Autodesk Inventor part; units mm, degrees
ref_plane "YZ Plane" through (0, 0, 0) normal (1, 0, 0) x (0, 1, 0)
ref_plane "XZ Plane" through (0, 0, 0) normal (0, 1, 0) x (-1, 0, 0)
ref_plane "XY Plane" through (0, 0, 0) normal (0, 0, 1) x (1, 0, 0)
sketch "Skizze1" plane through (0, 0, 0) normal (0, 0, 1) x (1, 0, 0)
  line L0 (16.6415, 9.8457) -> (8.5751, 9.8457)
  line L1 (8.5751, 9.8457) -> (8.5751, -9.8457)
  line L2 (8.5751, -9.8457) -> (16.6415, -9.8457)
  line L3 (16.6415, -9.8457) -> (16.6415, 9.8457)
  line L4 (16.6415, 9.8457) -> (8.5751, -9.8457) construction
  line L5 (8.5751, 9.8457) -> (16.6415, -9.8457) construction
  circle A0 centre (12.6083, 0) radius 2.6
  point P0 (0, 0)
  dimension "d0" = 5.2
extrude "Extrusion1" add sketch "Skizze1" along normal blind 3
sketch "Skizze2" plane through (0, 0, 3) normal (0, 0, 1) x (1, 0, 0)
  circle A0 centre (12.6083, 0) radius 2.6 construction
  line L0 (16.6415, 9.8457) -> (8.5751, 9.8457) construction
  line L1 (8.5751, 9.8457) -> (8.5751, -9.8457) construction
  line L2 (8.5751, -9.8457) -> (16.6415, -9.8457) construction
  line L3 (16.6415, -9.8457) -> (16.6415, 9.8457) construction
  line L4 (8.5751, 9.8457) -> (8.5751, -9.8457)
  line L5 (16.6415, -9.8457) -> (8.5751, -9.8457)
  line L6 (8.5751, -9.8457) -> (8.5751, -6.7929)
  line L7 (8.5751, -6.7929) -> (16.6415, -6.7929)
  line L8 (16.6415, -6.7929) -> (16.6415, -9.8457)
  line L9 (16.6415, -9.8457) -> (16.6415, 9.8457)
  line L10 (8.5751, 9.8457) -> (16.6415, 9.8457)
  line L11 (16.6415, 9.8457) -> (16.6415, 7.3365)
  line L12 (16.6415, 7.3365) -> (8.5751, 7.3365)
  line L13 (8.5751, 7.3365) -> (8.5751, 9.8457)
  point P0 (0, 0)
extrude "Extrusion2" add sketch "Skizze2" along normal blind 25 contours L10 L9 L12 L4 | L7 L8 L5 L4
sketch "Skizze3" plane through (8.5751, 7.3365, 3) normal (0, -1, 0) x (1, 0, 0)
  line L0 (8.0665, 0) -> (0, 0)
  line L1 (8.0665, 0) -> (8.0665, 25)
  line L2 (0, 25) -> (8.0665, 25)
  line L3 (0, 0) -> (0, 25)
  circle A0 centre (4.0332, 20.469) radius 1.4552
  point P0 (-8.5751, -3)
extrude "Extrusion3" cut sketch "Skizze3" along normal through all both and the other way through all contours A0
sketch "Skizze4" plane through (8.5751, -9.8457, 0) normal (0, -1, 0) x (1, 0, 0)
  line L0 (8.0665, 3) -> (8.0665, 28)
  line L1 (0, 3) -> (0, 28)
  line L2 (8.0665, 28) -> (0, 28)
  line L3 (0, 28) -> (0, 26.1511)
  line L4 (0, 26.1511) -> (8.0665, 26.1511)
  line L5 (8.0665, 26.1511) -> (8.0665, 28)
  point P0 (-8.5751, 0)
extrude "Extrusion4" cut sketch "Skizze4" against normal through all
sketch "Skizze5" plane through (16.6415, -9.8457, 0) normal (1, 0, 0) x (0, 0, -1)
  ellipse E0 centre (-12.9855, 10.4116) end of major axis (-22.9331, 10.4116) minor radius 7.8919
  point P0 (0, 9.8457)
extrude "Extrusion5" cut sketch "Skizze5" along normal through all both and the other way through all
properties part number "amt_dragster"
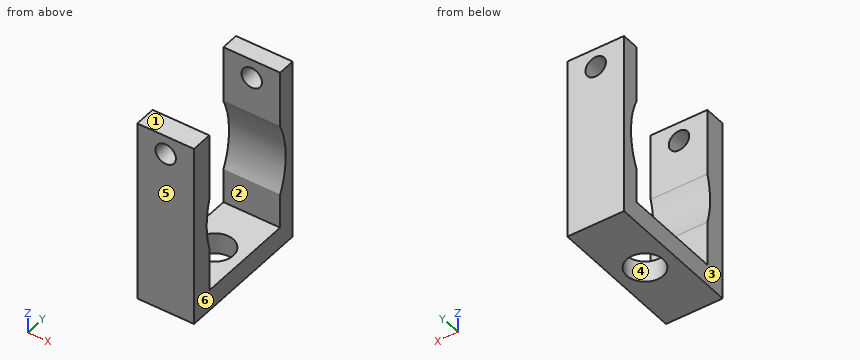
Work out the finished part from the listing and answer in its coordinate system (mm). Face numbers are marked on the shaded views. A direction names the side the tool comes from. Round coordinates to 2 decimals unless told otherwise and drop trailing zeros. Order: outer loops, then holes, each group sorted by start corner. A loop starts at its lowest first (then second) coordinate and runs counter-clockwise, first axis right, second up.
Q1. The mould has two halves that part along X. Classify the marked faces 3, 4, 5 and 6: pulls with the +X half, pulls with the -X half, needs draft (parallel to the pull), parting line crosses it, or undercut.
Solution:
face 3: pulls with the -X half
face 4: undercut
face 5: needs draft
face 6: pulls with the +X half
Q2. A tool of negligible diameter and unlimited length cuts with its end or side. For the marked faces 1 and 2, from which of +Z, -Z, +X, -X, +Y, -Y can it reach the whole face along a straight path? Write none if from no direction.
Solution:
face 1: +Z, +X, -X, +Y, -Y
face 2: +Z, +X, -X
Q3. A cutting plane is placed at C-C, the plane y = 8. Count the separate pieces of the cut face and the enclosed holes in it, then the cut area to 3 significant figures.
Solution:
separate pieces: 2
enclosed holes: 1
area: 150 mm2
Q4. Given pin 1 Ø4 at (x, y) = (12.61, 0) entering from +Z; pin 2 Ø2.5 at (x, y) = (14, -3) entering from +Z, each flat-ended and moving along its own axis, determine where each tip first touches the part or whether it passes through.
Solution:
pin 1: passes through
pin 2: stops at z = 3
Q5. Find the intervals of material crossed by line 1 along Y through (x, z) = (15, 22); line 2 along Z through (x, y) = (11.25, -4.25); line 3 along Z through (x, y) = (12, -7.5), in increasing order.
Solution:
line 1: y = -9.85 to -6.79, 7.34 to 9.85
line 2: z = 0 to 3
line 3: z = 0 to 22.15, 24.79 to 26.15
Q6. A cutting plane is placed at B-B, the plane y = 0. Determine the outline of the cut face in (x, z), then the cut area to 3 significant figures.
Solution:
outline: (8.58, 0) - (10.01, 0) - (10.01, 3) - (8.58, 3) - close; (15.21, 0) - (16.64, 0) - (16.64, 3) - (15.21, 3) - close
area: 8.60 mm2
Q7. A cutting plane is placed at A-A, the plane z = 3.5. Determine the outline of the cut face in (x, y), then the cut area to 3 significant figures.
Solution:
outline: (8.58, -9.85) - (16.64, -9.85) - (16.64, -6.79) - (8.58, -6.79) - close; (8.58, 7.34) - (16.64, 7.34) - (16.64, 9.85) - (8.58, 9.85) - close
area: 44.9 mm2
